Drawing for the job (mm, zero at the part's lowest x, y, z). Coordinates: 2 decimals unless noted, no trailing zeros. Loops run counter-clockwise (first coordinate to the right, second up) from the corner with the lowest first, then second, coordinate; pieces in that order, holes last. Notation, with made-up numbers: (64.5, -14) - (82.5, -14) arc R14 ccw to (82.5, -7) - close; hole circle Ø1 at (88.5, 30.25). An arc over 180 degrees is marked (long way). One line per item, written item: value.
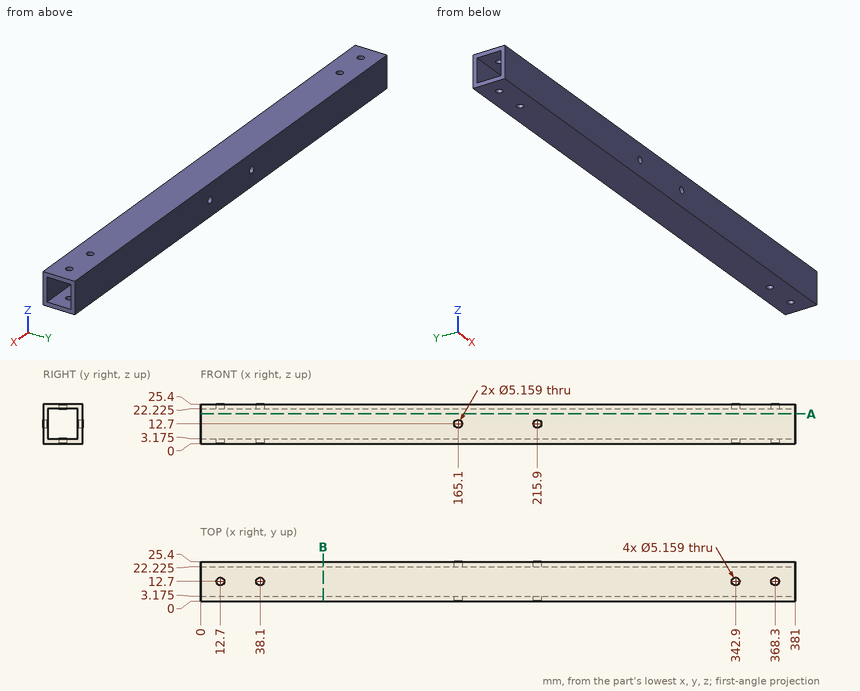
Item 1: Drop a flat-ended pin along its axis: P1, Ø4, axis at x = 368.3, y = 12.7, coming from the +Z side. Give the stop position or say it passes through.
Check result:
P1: passes through
Item 2: Probe probe 1 along X at (y, z) = (2.2, 12.7); probe 2 along Y at (x, z) = (38.1, 23.1); probe 3 along Y at (x, z) = (254.5, 7) (1 decimal). List the from-to ranges inside material, lowest first. Write a range as from..to.
Check result:
probe 1: x = 0..162.52, 167.68..213.32, 218.48..381
probe 2: y = 0..10.12, 15.28..25.4
probe 3: y = 0..3.2, 22.2..25.4
Item 3: Cut at A-A, the plane z = 19. Write the cut outline in (x, y) (1 decimal), then the cut area to 3 significant figures.
Check result:
outline: (0, 0) - (381, 0) - (381, 3.2) - (0, 3.2) - close; (0, 22.2) - (381, 22.2) - (381, 25.4) - (0, 25.4) - close
area: 2,420 mm^2
Item 4: Cut at B-B, the plane x = 78.5. Write the cut outline in (y, z) (1 decimal).
Check result:
outline: (0, 0) - (25.4, 0) - (25.4, 25.4) - (0, 25.4) - close; hole (3.2, 3.2) - (22.2, 3.2) - (22.2, 22.2) - (3.2, 22.2) - close
